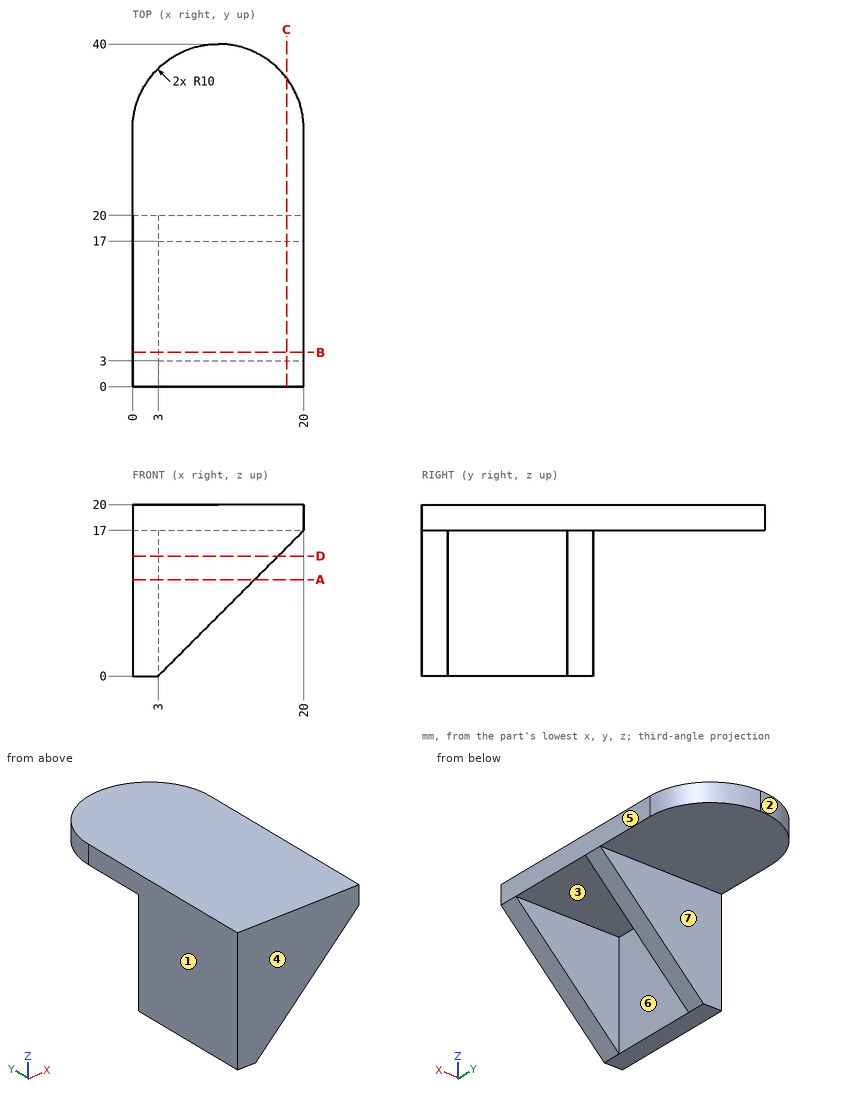
Geometry check sheet. Reference: drawing and pictorial views, mm from the part's lowest x, y, z. A direction names the side the tool comes from. Coordinates: 2 decimals unless noted, no trailing zeros. Write each loop counter-clockwise with the first axis right and the second up, starting at its lowest first coordinate (ties: lowest second). Pieces come first, ordered by that corner, then holes.
Item 1: Scan lines: probe 1 along Y at (x, z) = (8, 15.25); probe 2 along X at (y, z) = (8, 4.5); probe 3 along Z at (x, y) = (7.75, 36). Record each from-to range of solid material in increasing order.
Numbers:
probe 1: y = 0 to 3, 17 to 20
probe 2: x = 0 to 3
probe 3: z = 17 to 20
Item 2: Cross-section at B-B on y = 4. Record the boundary of the cut face in (x, z), then the cut area to 3 significant figures.
Numbers:
outline: (0, 0) - (3, 0) - (3, 17) - (20, 17) - (20, 20) - (0, 20) - close
area: 111 mm2
Item 3: Cross-section at C-C on x = 18. Record the boundary of the cut face in (y, z), then the cut area to 3 significant figures.
Numbers:
outline: (0, 15) - (3, 15) - (3, 17) - (17, 17) - (17, 15) - (20, 15) - (20, 17) - (36, 17) - (36, 20) - (0, 20) - close
area: 120 mm2
Item 4: Cross-section at D-D on z = 14. Record the boundary of the cut face in (x, y), then the cut area to 3 significant figures.
Numbers:
outline: (0, 0) - (17, 0) - (17, 3) - (3, 3) - (3, 17) - (17, 17) - (17, 20) - (0, 20) - close
area: 144 mm2
Item 5: Cross-section at A-A on z = 11.25. Record the boundary of the cut face in (x, y), then the cut area to 4 significant figures.
Numbers:
outline: (0, 0) - (14.25, 0) - (14.25, 3) - (3, 3) - (3, 17) - (14.25, 17) - (14.25, 20) - (0, 20) - close
area: 127.5 mm2
Item 6: Depth check by flat-ended pin: pin 1 Ø4 at (x, y) = (7.5, 7.5) entering from -Z; pin 2 Ø8 at (x, y) = (13.5, 16.5) entering from -Z; pin 3 Ø8.5 at (x, z) = (13.5, 12) entering from +Y. Enter the tip coordinate at first touch or a pass-through.
Numbers:
pin 1: stops at z = 17
pin 2: stops at z = 6.53
pin 3: stops at y = 20
Item 7: Mould release check, pull along Y, two halves, no side actions. Record for the marked faces 1, 2, 3 and 4: released by +Y, released by -Y, zero draft, split by the parting line, or undercut.
Numbers:
face 1: zero draft
face 2: released by +Y
face 3: undercut
face 4: released by -Y
Item 8: Access from +Z, -Z, +X, -X, +Y, -Y to the whole of each face (thin tool, end or side, straight path). Record for the marked faces 5, 6 and 7.
Numbers:
face 5: +Z, -Z, +X, +Y, -Y
face 6: -Z, +X
face 7: -Z, +X, -X, +Y
